The model under review builds one solid part; all positions refer to its coordinate system, in mm. Face numbers are marked on the shaded views. A direction names the side the tool comes from. Round coordinates to 2 decimals unless told otherwise and drop trailing zeros. Order: outer loops, then holes, each group sorted by start corner. A loop starts at its lowest first (then second) coordinate and runs counter-clockwise, first axis right, second up. Notation, with made-up numbers: M 82,28.5 L 130,28.5 A29 ccw 130,67.5 Z; hole C 20,-25.5 d2. An arc over 180 degrees is marked long. Answer as CSV lines item,"result". Start each with the question number.
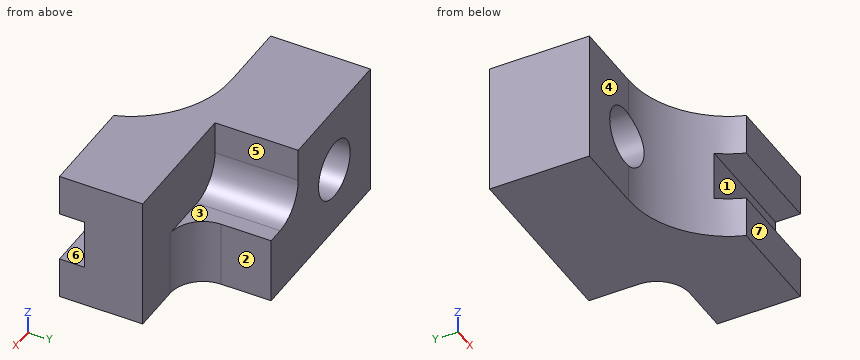
Autodesk Inventor part; units mm, degrees
ref_plane "YZ Plane" through (0, 0, 0) normal (1, 0, 0) x (0, 1, 0)
ref_plane "XZ Plane" through (0, 0, 0) normal (0, 1, 0) x (-1, 0, 0)
ref_plane "XY Plane" through (0, 0, 0) normal (0, 0, 1) x (1, 0, 0)
sketch "Sketch1" plane through (0, 0, 0) normal (0, 0, 1) x (1, 0, 0)
  line L0 (0, 0) -> (0, 76.2)
  line L1 (0, 76.2) -> (139.7, 76.2)
  line L2 (139.7, 76.2) -> (139.7, 38.1)
  line L3 (165.1, 12.7) -> (203.2, 12.7)
  line L4 (203.2, 12.7) -> (203.2, -50.8)
  line L5 (203.2, -50.8) -> (127, -50.8)
  line L6 (0, 0) -> (55.158, 0)
  arc A0 (139.7, 38.1) -> (165.1, 12.7) centre (165.1, 38.1) ccw
  arc A1 (127, -50.8) -> (55.158, 0) centre (55.158, -76.2) ccw
  dimension "d0" = 76.2
  dimension "d2" = 203.2
  dimension "d3" = 139.7
  dimension "d4" = 76.2
  dimension "d5" = 127
  dimension "d6" = 63.5
  dimension "d7" = 25.4
  dimension "d8" = 76.2
extrude "Extrusion1" add sketch "Sketch1" along normal blind 101.6
sketch "Sketch2" plane through (0, 76.2, 0) normal (0, 1, 0) x (1, 0, 0)
  line L0 (139.7, 0) -> (139.7, -50.8)
  line L1 (139.7, 0) -> (139.7, -101.6)
  line L2 (0, -101.6) -> (101.6, -101.6)
  line L3 (127, -101.6) -> (55.158, -101.6)
  line L4 (101.6, -101.6) -> (101.6, -76.2)
  line L5 (127, -50.8) -> (139.7, -50.8)
  arc A0 (127, -50.8) -> (101.6, -76.2) centre (127, -76.2) ccw
  line L6 (101.6, -101.6) -> (139.7, -101.6)
  line L7 (139.7, -101.6) -> (165.1, -101.6)
  line L8 (165.1, -101.6) -> (165.1, -50.8)
  line L9 (165.1, 0) -> (165.1, -101.6)
  line L10 (165.1, -50.8) -> (139.7, -50.8)
  point P0 (0, 0)
  dimension "d11" = 50.8
  dimension "d12" = 101.6
  dimension "d13" = 25.4
extrude "Extrusion3" cut sketch "Sketch2" against normal blind 63.5
sketch "Sketch3" plane through (0, 76.2, 0) normal (0, 1, 0) x (1, 0, 0)
  circle A0 centre (50.8, -50.8) radius 22.225
  line L0 (55.158, 0) -> (0, 0)
  line L1 (0, 0) -> (0, -101.6)
  dimension "d18" = 44.45
  dimension "d19" = 50.8
  dimension "d20" = 50.8
extrude "Extrusion4" cut sketch "Sketch3" against normal through all
sketch "Sketch4" plane through (203.2, -50.8, 0) normal (1, 0, 0) x (0, 0, -1)
  line L0 (0, 0) -> (-31.75, 0)
  line L1 (0, 0) -> (-101.6, 0)
  line L2 (-31.75, 0) -> (-31.75, 19.05)
  line L3 (-31.75, 19.05) -> (-69.85, 19.05)
  line L4 (-69.85, 19.05) -> (-69.85, 0)
  line L5 (-31.75, 0) -> (-69.85, 0)
  point P0 (0, 50.8)
  dimension "d23" = 31.75
  dimension "d24" = 19.05
  dimension "d25" = 38.1
extrude "Extrusion5" cut sketch "Sketch4" against normal through all
properties part number "HW 8 Part 1"
Item 1: Consider section B-B (z = 22.5). State the section outline as (x, y) points, and give its area (3 significant figures).
Item 2: Consider section C-C (y = 17.5). State the section outline as (x, z) points (3 decimals).
Item 3: Tool access review of the marked faces 4, 5, 6 and 7: name each direction out of +Z, -Z, +X, -X, +Y, -Y from which nothing blocks a thin tool from reaching the whole face with its end or side.
Item 4: For pin 1 (2 mm diameter, centred on y = 55.5, z = 47.5, fed in from -X); pin 2 (7.5 mm diameter, centred on y = 45, z = 88.5, fed in from +X); pin 3 (4 mm diameter, centred on x = 175, z = 30, fed in from +Y); pin 4 (3 mm diameter, centred on x = 104, z = 74.5, fed in from -Y), all flat-tipped, find the tip position at first contact; note any pin that passes through.
Item 5: Wall thickness on probe 1 along Z at (x, y) = (50, 44); probe 2 along Z at (x, y) = (147, -37); probe 3 along X at (y, z) = (52.5, 8.5): over which ranges is each line inside the solid? List them lowest first. Write a range as [from, to].
Item 6: Consider section A-A (x = 50.8). State the section outline as (y, z) points (3 decimals).
Item 7: The part is to be moulded in two halves that separate along Z. For the marked faces 1, 2 and 3, say which applies: +Z half, -Z half, draft (parallel to the pull), parting line (faces both ways), or undercut.
Item 8: Consider section D-D (y = -36.5). State the section outline as (x, z) points.
Reported:
1,outline,"M 0,0 L 55.16,0 A76.2 cw 127,-50.8 L 203.2,-50.8 L 203.2,12.7 L 165.1,12.7 A25.4 cw 139.7,38.1 L 139.7,76.2 L 0,76.2 Z"
1,area,"16,400 mm²"
2,outline,"M 0,0 L 150.241,0 L 150.241,50.8 L 127,50.8 A25.4 cw 101.6,76.2 L 101.6,101.6 L 0,101.6 Z; hole C 50.8,50.8 d44.45"
3,face 4,"+Z, -Z, -X, -Y"
3,face 5,"+Z, +X, +Y"
3,face 6,"+X, -X, -Y"
3,face 7,"+Z, -Z, +X, -X, -Y"
4,pin 1,"stops at x = 0"
4,pin 2,"stops at x = 101.6"
4,pin 3,"stops at y = 12.7"
4,pin 4,"stops at y = -19"
5,probe 1,"z = [0, 28.59], [73.01, 101.6]"
5,probe 2,"z = [0, 31.75], [69.85, 101.6]"
5,probe 3,"x = [0, 139.7]"
6,outline,"M 0,0 L 76.2,0 L 76.2,28.575 L 0,28.575 Z; M 0,73.025 L 76.2,73.025 L 76.2,101.6 L 0,101.6 Z"
7,face 1,"undercut"
7,face 2,"draft"
7,face 3,"+Z half"
8,outline,"M 120.2,0 L 203.2,0 L 203.2,31.75 L 120.2,31.75 Z; M 120.2,69.85 L 203.2,69.85 L 203.2,101.6 L 120.2,101.6 Z"
